from build123d import *

# Parameters (mm, degrees)
SKETCH_1_R          = 1.55
EXTRUDE_1_DEPTH     = 3
SKETCH_2_W          = 30.67898901
SKETCH_2_H          = 20.291672983
CUT_EXTRUDE_1_DEPTH = 10
SKETCH_3_R          = 1
CUT_EXTRUDE_2_DEPTH = 20
CUT_EXTRUDE_3_DEPTH = 100.15206986
FILLET_1_R          = 2


with BuildPart() as part:
    # 草图1 → 凸台-拉伸1 (new body)
    with BuildSketch(Plane.XY):
        with BuildLine():
            Line((5, 16.216737463), (-5, 16.216737463))
            ThreePointArc((-5, 16.216737463), (-7.121320344, 15.338057806), (-8, 13.216737463))
            Line((-8, 13.216737463), (-8, -66.783262537))
            Line((-8, -66.783262537), (-4, -108.783262537))
            Line((-4, -108.783262537), (4, -108.783262537))
            Line((4, -108.783262537), (8, -66.783262537))
            Line((8, -66.783262537), (8, 13.216737463))
            ThreePointArc((8, 13.216737463), (7.121320344, 15.338057806), (5, 16.216737463))
        make_face()
        with Locations((-4.949747468, 11.166484931)):
            Circle(SKETCH_1_R, mode=Mode.SUBTRACT)
        with Locations((4.949747468, 11.166484931)):
            Circle(SKETCH_1_R, mode=Mode.SUBTRACT)
        with Locations((4.949747468, 1.266989995)):
            Circle(SKETCH_1_R, mode=Mode.SUBTRACT)
        with Locations((-4.949747468, 1.266989995)):
            Circle(SKETCH_1_R, mode=Mode.SUBTRACT)
        with Locations((0, -43.783262537)):
            Circle(SKETCH_1_R, mode=Mode.SUBTRACT)
        with Locations((4.949747468, -38.833515069)):
            Circle(SKETCH_1_R, mode=Mode.SUBTRACT)
        with Locations((-4.949747468, -38.833515069)):
            Circle(SKETCH_1_R, mode=Mode.SUBTRACT)
        with Locations((4.949747468, -48.733010005)):
            Circle(SKETCH_1_R, mode=Mode.SUBTRACT)
        with Locations((-4.949747468, -48.733010005)):
            Circle(SKETCH_1_R, mode=Mode.SUBTRACT)
        with Locations((0, 6.216737463)):
            Circle(SKETCH_1_R, mode=Mode.SUBTRACT)
    extrude(amount=EXTRUDE_1_DEPTH)

    # 草图2 → 切除-拉伸1 (cut)
    with BuildSketch(Plane(origin=(0, 0, 0), x_dir=(-1, 0, 0), z_dir=(0, 0, -1))):
        with Locations((1.230440634, -108.929099029)):
            Rectangle(SKETCH_2_W, SKETCH_2_H)
    extrude(amount=-CUT_EXTRUDE_1_DEPTH, mode=Mode.SUBTRACT)

    # 草图3 → 切除-拉伸2 (cut)
    with BuildSketch(Plane(origin=(0, 0, 0), x_dir=(-1, 0, 0), z_dir=(0, 0, -1))):
        with Locations((0, -83.783262537)):
            Circle(SKETCH_3_R)
        with Locations((0, -90.783262537)):
            Circle(SKETCH_3_R)
        with Locations((0, -73.783262537)):
            Circle(SKETCH_3_R)
    extrude(amount=-CUT_EXTRUDE_2_DEPTH, mode=Mode.SUBTRACT)

    # 草图4 → 切除-拉伸3 (cut, through all)
    with BuildSketch(Plane(origin=(0, 0, 0), x_dir=(-1, 0, 0), z_dir=(0, 0, -1))):
        Polygon((6, -12.783262537), (-6, -30.783262537), (-6, -33.833515069), (6, -33.833515069), align=None)
        Polygon((6, -3.733010005), (-6, -3.733010005), (-6, -24.783262537), (6, -6.783262537), align=None)
        Polygon((6, -66.783262537), (6, -53.976503319), (-2.537839478, -66.783262537), align=None)
        Polygon((-6, -65.976503319), (2.537839478, -53.169744102), (-6, -53.169744102), align=None)
    extrude(amount=-CUT_EXTRUDE_3_DEPTH, mode=Mode.SUBTRACT)

    # 圆角1
    fillet_1_edges = [part.edges().sort_by_distance(p)[0] for p in [
        (6, -30.783262537, 1.5),
        (-6, -12.783262537, 1.5),
        (-6, -33.833515069, 1.5),
        (6, -33.833515069, 1.5),
        (-2.537839478, -53.169744102, 1.5),
        (6, -65.976503319, 1.5),
        (6, -53.169744102, 1.5),
        (-6, -53.976503319, 1.5),
        (-6, -66.783262537, 1.5),
        (2.537839478, -66.783262537, 1.5),
        (6, -24.783262537, 1.5),
        (6, -3.733010005, 1.5),
        (-6, -3.733010005, 1.5),
        (-6, -6.783262537, 1.5),
    ]]
    fillet(fillet_1_edges, radius=FILLET_1_R)


solid = part.part
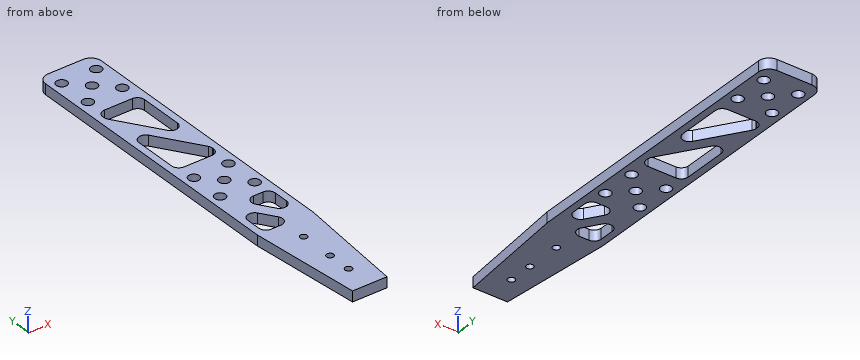
Verification items for the finished model (mm, model axes). Give positions to 0.01 mm unless a question says otherwise; leave off trailing zeros. Write each loop counter-clockwise with the first axis right and the second up, starting at its lowest first coordinate (ties: lowest second). Pieces come first, ordered by that corner, then holes.
(1) Cross-section at A-A (y = -15). Enter the section's corners in (x, z).
(2) Cross-section at B-B (z = 0.55). State how many separate pieces and enclosed holes the cut face has, plus the area to 3 significant figures.
(3) Material ranges on line 1 (X direction, y = -18, z = 0.6); line 2 (X direction, y = 10, z = 2.7); line 3 (X direction, y = 6, z = 2.4), recorded low to high.
Worked out:
1. outline: (-8, 0) - (-0.52, 0) - (-0.52, 3) - (-8, 3) - close; (6, 0) - (8, 0) - (8, 3) - (6, 3) - close
2. separate pieces: 1
2. enclosed holes: 17
2. area: 1,300 mm2
3. line 1: x = -8 to -5.44, -2.56 to 1.48, 6 to 8
3. line 2: x = -8 to -5.97, -3.93 to 3.93, 5.97 to 8
3. line 3: x = -8 to -1.53, 1.53 to 8
